Could you check a few things on this model? Use its own coordinates, in mm. Face numbers are marked on the shaded views. A direction names the side the tool comes from. Round coordinates to 2 decimals unless told otherwise and drop trailing zeros. Write each loop counter-clockwise with the first axis right and the second up, starting at its lowest first coordinate (ties: lowest second). Pieces come first, ordered by that corner, then holes. Notation, with made-up numbers: (-6.75, -11) -> (50.25, -11) arc R9 cw to (50.25, 6) -> close; hole circle Ø8 at (25, 57.5). An arc over 180 degrees is marked (long way). Answer in a Markdown table with one row per item.
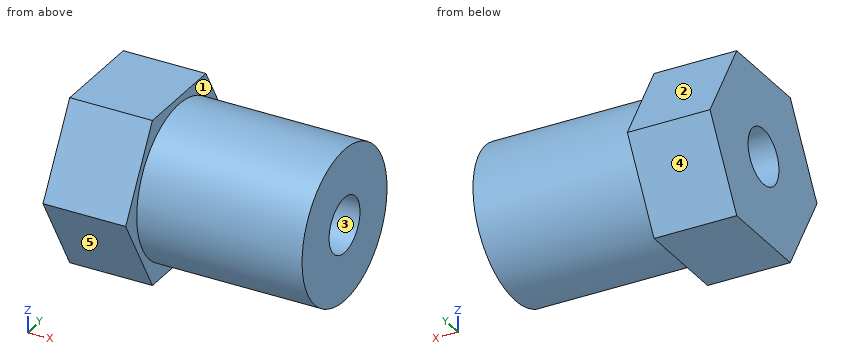
Autodesk Inventor part; units mm, degrees
ref_plane "YZ Plane" through (0, 0, 0) normal (1, 0, 0) x (0, 1, 0)
ref_plane "XZ Plane" through (0, 0, 0) normal (0, 1, 0) x (-1, 0, 0)
ref_plane "XY Plane" through (0, 0, 0) normal (0, 0, 1) x (1, 0, 0)
sketch "Skizze1" plane through (0, 0, 0) normal (1, 0, 0) x (0, 1, 0)
  line L0 (6.9282, 0) -> (3.4641, -6)
  line L1 (3.4641, -6) -> (-3.4641, -6)
  line L2 (-3.4641, -6) -> (-6.9282, 0)
  line L3 (-6.9282, 0) -> (-3.4641, 6)
  line L4 (-3.4641, 6) -> (3.4641, 6)
  line L5 (3.4641, 6) -> (6.9282, 0)
  point P0 (0, 0)
  point P1 (0, 0)
  dimension "d0" = 12
extrude "Extrusion1" add sketch "Skizze1" along normal blind 6
sketch "Skizze2" plane through (6, 0, 0) normal (1, 0, 0) x (0, 0, -1)
  circle A0 centre (0, 0) radius 5.5
  dimension "d3" = 11
extrude "Extrusion2" add sketch "Skizze2" along normal blind 12
sketch "Skizze3" plane through (18, 0, 0) normal (1, 0, 0) x (0, 0, -1)
  circle A0 centre (0, 0) radius 2
  dimension "d6" = 4
extrude "Extrusion3" cut sketch "Skizze3" against normal through all
properties part number "MotorAdapter"
1) Imagine slicing it at A-A, the plane y = 0. Please give me the cut outline in (x, z), plus the area to 3 significant figures.
Findings:
| item | result |
|---|---|
| outline | (0, -6) -> (6, -6) -> (6, -5.5) -> (18, -5.5) -> (18, -2) -> (0, -2) -> close; (0, 2) -> (18, 2) -> (18, 5.5) -> (6, 5.5) -> (6, 6) -> (0, 6) -> close |
| area | 132 mm^2 |
2) For the marked faces 1 and 2, which set-ups out of +Z, -Z, +X, -X, +Y, -Y let a thin tool reach every point of the face, with its end or its side?
Findings:
| item | result |
|---|---|
| face 1 | +X |
| face 2 | +Z, +X, -X, +Y |
3) Thinking about a two-plate mould opening in Y: for the marked faces 3, 4 and 5, which applies, +Y half, -Y half, draft (parallel to the pull), parting line (faces both ways), or undercut?
Findings:
| item | result |
|---|---|
| face 3 | undercut |
| face 4 | +Y half |
| face 5 | -Y half |
4) For pin 1 (4.5 mm diameter, centred on y = 0, z = 0, fed in from +X); pin 2 (1 mm diameter, centred on y = -5, z = 4.5, fed in from +X); pin 3 (6 mm diameter, centred on x = 10.5, z = 2, fed in from +Y); pin 4 (1 mm diameter, centred on x = 9.5, z = 0, fed in from -Y), each with a flat end and sliding along its axis, tell me the tip position at first contact or that it passes through.
Findings:
| item | result |
|---|---|
| pin 1 | stops at x = 18 |
| pin 2 | passes through |
| pin 3 | stops at y = 5.5 |
| pin 4 | stops at y = -5.5 |
5) Imagine slicing it at C-C, the plane z = 1.25. Please give me the cut outline in (x, y), plus the area to 3 significant figures.
Findings:
| item | result |
|---|---|
| outline | (0, -6.21) -> (6, -6.21) -> (6, -5.36) -> (18, -5.36) -> (18, -1.56) -> (0, -1.56) -> close; (0, 1.56) -> (18, 1.56) -> (18, 5.36) -> (6, 5.36) -> (6, 6.21) -> (0, 6.21) -> close |
| area | 147 mm^2 |
6) Imagine slicing it at B-B, the plane x = 2.75. Please give me the cut outline in (y, z).
Findings:
| item | result |
|---|---|
| outline | (-6.93, 0) -> (-3.46, -6) -> (3.46, -6) -> (6.93, 0) -> (3.46, 6) -> (-3.46, 6) -> close; hole circle Ø4 at (0, 0) |
7) Please list where these lines run through material, in increasing order: line 1 (Y direction, x = 13.75, z = 0); line 2 (Z direction, x = 7.75, y = -1.5); line 3 (Z direction, x = 16, y = -1).
Findings:
| item | result |
|---|---|
| line 1 | y = -5.5 to -2, 2 to 5.5 |
| line 2 | z = -5.29 to -1.32, 1.32 to 5.29 |
| line 3 | z = -5.41 to -1.73, 1.73 to 5.41 |
8) Imagine slicing it at D-D, the plane y = -4.5. Please give me the cut outline in (x, z), plus the area to 3 significant figures.
Findings:
| item | result |
|---|---|
| outline | (0, -4.21) -> (6, -4.21) -> (6, -3.16) -> (18, -3.16) -> (18, 3.16) -> (6, 3.16) -> (6, 4.21) -> (0, 4.21) -> close |
| area | 126 mm^2 |
